The listing builds one solid part. Answer for the finished solid, in the listing's coordinates (mm). A direction names the side the tool comes from. Round coordinates to 2 decimals unless told otherwise and drop trailing zeros. Loops run counter-clockwise (first coordinate to the right, second up) from the corner with the lowest first, then second, coordinate; pieces in that order, holes last. Notation, with made-up numbers: M 42.5,66.25 L 48.5,66.25 A15 cw 48.5,95.25 Z; hole C 50,29 d1. An arc over 180 degrees is marked long. Answer as a JSON object with one key per item and string values.
```python
from build123d import *

# Parameters (mm, degrees)
SKETCH1_R           = 3.175
SKETCH1_W           = 8.89
SKETCH1_H           = 4.953
BOSS_EXTRUDE1_DEPTH = 2.4765


with BuildPart() as part:
    # Sketch1 → Boss-Extrude1 (new, symmetric)
    with BuildSketch(Plane(origin=(0, 0, 0), x_dir=(1, 0, 0), z_dir=(0, 1, 0))):
        with BuildLine():
            Line((30.607, -21.59), (30.607, 5.08))
            Line((30.607, 5.08), (35.052, 5.08))
            Line((35.052, 5.08), (35.052, 12.7))
            Line((35.052, 12.7), (0.169883273, 12.7))
            ThreePointArc((0.169883273, 12.7), (-6.518875251, 10.18762116), (-9.899622874, 3.893013664))
            ThreePointArc((-9.899622874, 3.893013664), (-3.310755736, -18.802646574), (17.907, -29.21))
            Line((17.907, -29.21), (35.052, -29.21))
            Line((35.052, -29.21), (35.052, -21.59))
            Line((35.052, -21.59), (30.607, -21.59))
        make_face()
        Circle(SKETCH1_R, mode=Mode.SUBTRACT)
        with Locations((9.652, -15.24)):
            Rectangle(SKETCH1_W, SKETCH1_H, mode=Mode.SUBTRACT)
    extrude(amount=BOSS_EXTRUDE1_DEPTH, both=True)


solid = part.part
```
Item 1: Determine the mould class of faces 4 (the face through (26, 0, 29.21)), 5 (the face through (18, 0, -12.7)), 6 (the face through (5.207, 0, 15)), 7 (the face through (10, 0, 12.764)) for opening direction Z: released by +Z, released by -Z, zero draft, split by the parting line, or undercut.
Values follow:
{"face 4": "released by +Z", "face 5": "released by -Z", "face 6": "undercut", "face 7": "undercut"}
Item 2: The part is cut by section D-D (z = 24). Give the vertices of the cut face in (x, y).
Values follow:
{"outline": "M 2.38,-2.48 L 35.05,-2.48 L 35.05,2.48 L 2.38,2.48 Z"}
Item 3: The part is cut by section C-C (x = 7). Give the vertices of the cut face in (y, z).
Values follow:
{"outline": "M -2.48,-12.7 L 2.48,-12.7 L 2.48,12.76 L -2.48,12.76 Z; M -2.48,17.72 L 2.48,17.72 L 2.48,26.62 L -2.48,26.62 Z"}
Item 4: Straight lines are drawn through the part: line 1 (X direction, y = -0.1, z = 0) (3 decimals); line 2 (Z direction, x = 33, y = -0.7); line 3 (Z direction, x = 0, y = -0.6) (3 decimals). For each, find the intervals that lie inside material, in ascending order.
Values follow:
{"line 1": "-10.16 to -3.175, 3.175 to 30.607", "line 2": "-12.7 to -5.08, 21.59 to 29.21", "line 3": "-12.699 to -3.175, 3.175 to 22.154"}
Item 5: Flat-ended cylindrical pins translate along their axes: P1, Ø2, axis at y = -1.5, z = -5, coming from the -X side; P2, Ø2, axis at y = 2, z = 18.5, coming from the -X side. Find the tip coordinate at first contact, or state that the pin passes through.
Values follow:
{"P1": "x = -9.88", "P2": "x = -4.34"}
Item 6: Which of the six approach directions +Z, -Z, +X, -X, +Y, -Y give full straight-line access (tool end or side, diameter ignored) to faces 1 (the face through (30.607, 0, 8)), 2 (the face through (10, 0, 17.716)), 3 (the face through (-6.442, 0.035, -10.255))?
Values follow:
{"face 1": "+X, +Y, -Y", "face 2": "+Y, -Y", "face 3": "-Z, -X, +Y, -Y"}
Item 7: The part is cut by section B-B (y = 1.2). Give the number of separate pieces and of enclosed holes in the cut face, then the cut area to 3 significant figures.
Values follow:
{"separate pieces": "1", "enclosed holes": "2", "area": "1,490 mm^2"}
Item 8: The part is cut by section A-A (z = 0). Give the vertices of the cut face in (x, y) (1 decimal).
Values follow:
{"outline": "M -10.2,-2.5 L -3.2,-2.5 L -3.2,2.5 L -10.2,2.5 Z; M 3.2,-2.5 L 30.6,-2.5 L 30.6,2.5 L 3.2,2.5 Z"}
